```python
from build123d import *

# Parameters (mm, degrees)
SKETCH1_W           = 37
SKETCH1_H           = 37
BOSS_EXTRUDE1_DEPTH = 1260
SKETCH2_W           = 23.9
SKETCH2_H           = 40
CUT_EXTRUDE1_DEPTH  = 20
SKETCH3_W           = 23.9
SKETCH3_H           = 1.6
CUT_EXTRUDE2_DEPTH  = 20
CUT_EXTRUDE3_DEPTH  = 20
SKETCH5_W           = 4
SKETCH5_H           = 10
CUT_EXTRUDE4_DEPTH  = 10
LPATTERN1_COUNT     = 2
LPATTERN1_PITCH     = 400
SKETCH6_R           = 3
CUT_EXTRUDE5_DEPTH  = 1262.269202034


with BuildPart() as part:
    # Sketch1 → Boss-Extrude1 (new body)
    with BuildSketch(Plane(origin=(0, 0, 0), x_dir=(1, 0, 0), z_dir=(0, 1, 0))):
        with BuildLine():
            Line((0.5, 0), (39.5, 0))
            ThreePointArc((39.5, 0), (39.853553391, 0.146446609), (40, 0.5))
            Line((40, 0.5), (40, 39.5))
            ThreePointArc((40, 39.5), (39.853553391, 39.853553391), (39.5, 40))
            Line((39.5, 40), (0.5, 40))
            ThreePointArc((0.5, 40), (0.146446609, 39.853553391), (0, 39.5))
            Line((0, 39.5), (0, 0.5))
            ThreePointArc((0, 0.5), (0.146446609, 0.146446609), (0.5, 0))
        make_face()
        with Locations((20, 20)):
            Rectangle(SKETCH1_W, SKETCH1_H, mode=Mode.SUBTRACT)
    extrude(amount=BOSS_EXTRUDE1_DEPTH)

    # Sketch2 → Cut-Extrude1 (cut)
    with BuildSketch(Plane.XY):
        with Locations((20.05, 1240)):
            Rectangle(SKETCH2_W, SKETCH2_H)
    cut_extrude1 = extrude(amount=-CUT_EXTRUDE1_DEPTH, mode=Mode.SUBTRACT)

    # Sketch3 → Cut-Extrude2 (cut)
    with BuildSketch(Plane.XY.offset(-38.5)):
        with Locations((20.05, 1259.2)):
            Rectangle(SKETCH3_W, SKETCH3_H)
        with Locations((20.05, 1220.8)):
            Rectangle(SKETCH3_W, SKETCH3_H)
    cut_extrude2 = extrude(amount=-CUT_EXTRUDE2_DEPTH, mode=Mode.SUBTRACT)

    # Mirror1: Cut-Extrude1, Cut-Extrude2 across plane
    add(cut_extrude1.mirror(Plane.ZX.offset(630)), mode=Mode.SUBTRACT)
    add(cut_extrude2.mirror(Plane.ZX.offset(630)), mode=Mode.SUBTRACT)

    # Sketch4 → Cut-Extrude3 (cut)
    with BuildSketch(Plane(origin=(40, 0, 0), x_dir=(0, 0, -1), z_dir=(1, 0, 0))):
        Polygon((0, 840), (16.5, 840), (16.5, 820), (0, 820), (0, 825), (5, 825), (5, 835), (0, 835), align=None)
    cut_extrude3 = extrude(amount=-CUT_EXTRUDE3_DEPTH, mode=Mode.SUBTRACT)

    # Sketch5 → Cut-Extrude4 (cut)
    with BuildSketch(Plane.XY):
        with Locations((38, 830)):
            Rectangle(SKETCH5_W, SKETCH5_H)
    cut_extrude4 = extrude(amount=-CUT_EXTRUDE4_DEPTH, mode=Mode.SUBTRACT)

    # LPattern1: Cut-Extrude3, Cut-Extrude4 ×2
    with Locations(*[(0, -i * LPATTERN1_PITCH, 0) for i in range(1, LPATTERN1_COUNT)]):
        add(cut_extrude3, mode=Mode.SUBTRACT)
        add(cut_extrude4, mode=Mode.SUBTRACT)

    # Sketch6 → Cut-Extrude5 (cut, through all)
    with BuildSketch(Plane(origin=(40, 0, 0), x_dir=(0, 0, -1), z_dir=(1, 0, 0))):
        with Locations((20, 1140)):
            Circle(SKETCH6_R)
        with Locations((20, 120)):
            Circle(SKETCH6_R)
    extrude(amount=-CUT_EXTRUDE5_DEPTH, mode=Mode.SUBTRACT)


solid = part.part
```
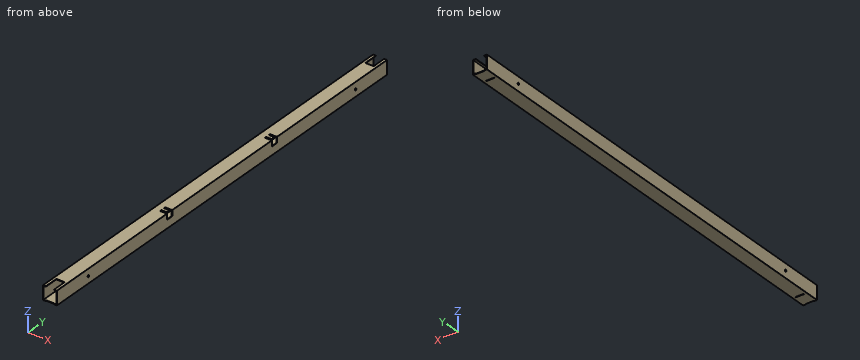
Build history of the part. All positions in model axes, mm. Round coordinates to 2 decimals unless told otherwise and drop trailing zeros. Loops run counter-clockwise (first coordinate to the right, second up) from the corner with the lowest first, then second, coordinate; pieces in that order, holes last.
Item 1: Saw through at A-A (z = -9.5). List the corners of the cut face in (x, y).
Item 2: Drill centre lines: line 1 along X through (y, z) = (863.5, -38); line 2 along Z through (x, y) = (9, 637); line 3 along Y through (x, z) = (39, -20). Where is each one in solid material? Low to high.
Item 3: Pin check, flat tips, straight feed: P1, Ø7, axis at y = 120, z = -20, coming from the +X side; P2, Ø0.8, axis at x = 15.5, z = -39, coming from the -Y side; P3, Ø1.6, axis at x = 19, z = -39.5, coming from the +Y side. Stop position of each tip, or through.
Worked answers:
1. outline: (0, 0) - (1.5, 0) - (1.5, 1260) - (0, 1260) - close; (38.5, 0) - (40, 0) - (40, 420) - (38.5, 420) - close; (38.5, 440) - (40, 440) - (40, 820) - (38.5, 820) - close; (38.5, 840) - (40, 840) - (40, 1260) - (38.5, 1260) - close
2. line 1: x = 0 to 1.5, 38.5 to 40
2. line 2: z = -40 to -38.5, -1.5 to 0
2. line 3: y = 0 to 117, 123 to 1137, 1143 to 1260
3. P1: stops at x = 40
3. P2: stops at y = 1.6
3. P3: stops at y = 1258.4
